Drawing for the job (mm, zero at the part's lowest x, y, z). A direction names the side the tool comes from. Coordinates: 2 decimals unless noted, no trailing zeros. Write each loop counter-clockwise with the first axis right and the second up, starting at its lowest first coordinate (ties: lowest second). Pieces come first, ordered by that corner, then holes. Notation, with made-up numbers: (85, 29.5) -> (136, 29.5) arc R9 ccw to (136, 37.5) -> close; hole circle Ø4 at (69, 20). An arc over 180 degrees is marked (long way). Answer as CSV lines item,"result". Start each with the question number.
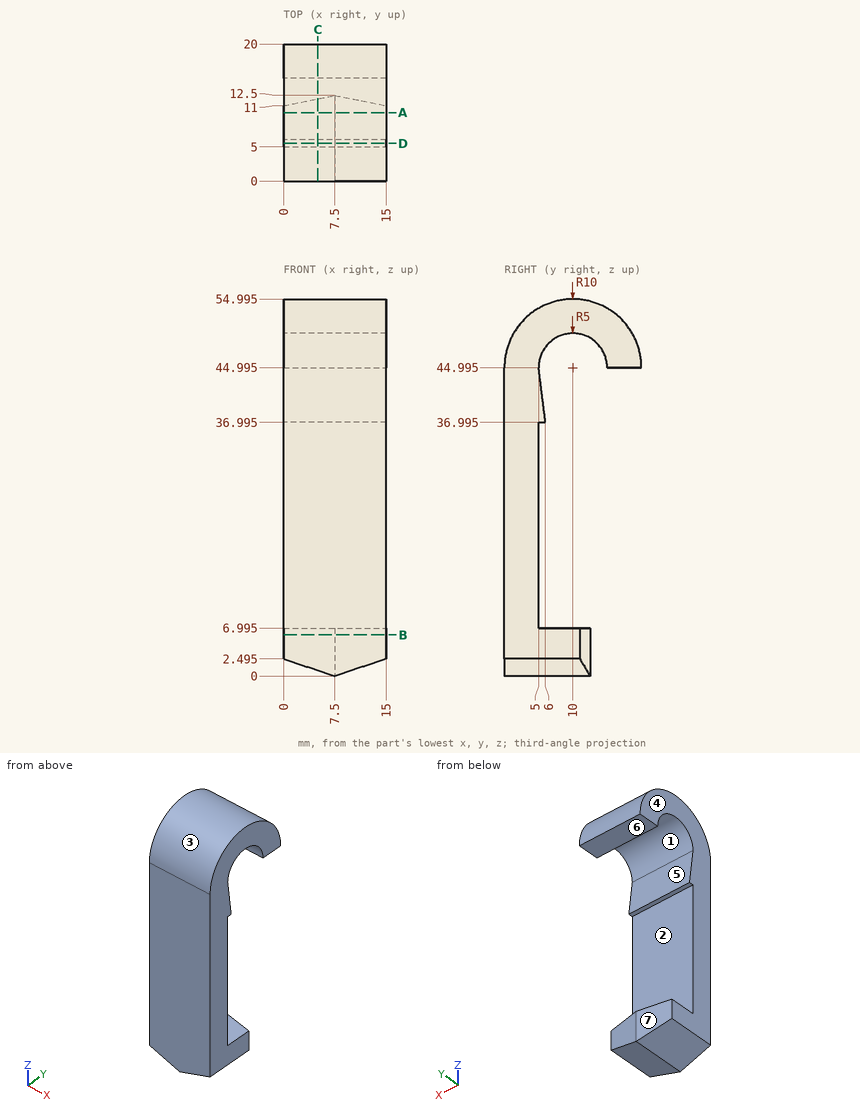
1. Cut at D-D (y = 5.5). Give the cut face in (x, z) (1 decimal).
2. Flat gauge pins, fed straight in: P1, Ø1, axis at x = 13.5, z = 41.5, coming from the +Y side; P2, Ø1.1, axis at x = 4, y = 5.5, coming from the -Z side; P3, Ø1, axis at x = 9, y = 7.5, coming from the +Z side. Where does each tip first touch, or does it go through?
3. Cut at A-A (y = 10). Give the cut face in (x, z) (3 decimals), then the cut area to 3 significant figures.
4. Wall check: line 1 (Y direction, x = 10.75, z = 23); line 2 (Z direction, x = 11.25, y = 11.5) (1 decimal); line 3 (Z direction, x = 2.5, y = 9) (1 decimal). Give the ranges that are in metal, low to high.
5. Mould opens along Z. For the marked faces 1, 2, 3 and 4 say: pulls with the +Z half, pulls with the -Z half, needs draft (parallel to the pull), parting line crosses it, or undercut.
6. Cut at B-B (z = 6). Give the cut face in (x, y).
7. Tool access for the marked faces 5, 6 and 7: list every direction of +Z, -Z, +X, -X, +Y, -Y with a clear straight run to the whole face (end or side of a thin tool).
8. Cut at C-C (x = 5). Give the cut face in (y, z) (1 decimal).
Geometry check:
1,outline,"(0, 2.5) -> (7.5, 0) -> (15, 2.5) -> (15, 7) -> (0, 7) -> close; (0, 37) -> (15, 37) -> (15, 41) -> (0, 41) -> close; (0, 47.2) -> (15, 47.2) -> (15, 53.9) -> (0, 53.9) -> close"
2,P1,"y = 5.5"
2,P2,"z = 0.98"
2,P3,"z = 54.79"
3,outline,"(0, 2.495) -> (7.5, 0) -> (15, 2.495) -> (15, 6.995) -> (0, 6.995) -> close; (0, 49.995) -> (15, 49.995) -> (15, 54.995) -> (0, 54.995) -> close"
3,area,"161 mm²"
4,line 1,"0 to 5"
4,line 2,"1.2 to 7, 49.8 to 54.9"
4,line 3,"1.7 to 7, 49.9 to 54.9"
5,face 1,"undercut"
5,face 2,"undercut"
5,face 3,"pulls with the +Z half"
5,face 4,"needs draft"
6,outline,"(0, 0) -> (15, 0) -> (15, 11) -> (7.5, 12.5) -> (0, 11) -> close"
7,face 5,"+X, -X, +Y"
7,face 6,"-Z, +X, -X, +Y"
7,face 7,"-Z, -X, +Y"
8,outline,"(0, 0.8) -> (12, 0.8) -> (12, 7) -> (5, 7) -> (5, 37) -> (6, 37) -> (5, 45) arc R5 cw to (15, 45) -> (20, 45) arc R10 ccw to (0, 45) -> close"
